Read the model definition and answer for the solid it produces. Units are mm, in the model's axes. A direction names the side the tool comes from. Round coordinates to 2 decimals unless told otherwise and drop trailing zeros. Write each loop counter-clockwise with the first axis right and the second up, starting at its lowest first coordinate (ties: lowest second). Pieces come first, ordered by that corner, then holes. Notation, with made-up numbers: (31.5, 46.25) - (73.5, 46.25) arc R27 cw to (73.5, 81.25) - close; hole circle Ø10 at (43, 33.5). An arc over 180 degrees is marked (long way). Answer as CSV lines item,"result". Start each with the question number.
1) For a pull along Y with two mould halves and no side action, classify faces 4 (the flat face through (-16, -10, 0)), 5 (the flat face through (6.736, 6.267, 1.972)), 6 (the cylindrical face through (-62, 36.12, 17.97)), 7 (the flat face through (-0.946, -35.738, 1.972)) as +Y half, -Y half, draft (parallel to the pull), parting line (faces both ways), or undercut.
2) Find section C-C on x = -38. Determine the outline of the cut face in (y, z).
3) Consider line 1 along X through (y, z) = (17.5, 2.5); line 2 along X through (y, z) = (-19, 1.25); line 3 along X through (y, z) = (-10.5, 5.5). Determine where each line is inside the solid, lowest interval first.
4) Each of these flat-tipped pins is pushed along its axis until it touches: pin 1 (2.5 mm diameter, centred on x = -59.5, y = 28, fed in from -Z); pin 2 (1.5 mm diameter, centred on x = 28, y = 26.5, fed in from -Z); pin 3 (4 mm diameter, centred on x = -25.5, z = 16.5, fed in from -Y); pin 4 (5 mm diameter, centred on x = -11.5, z = 12.5, fed in from -Y). Where does it stop, or does it pass through?
5) Find section A-A on z = 18.5. Determine the outline of the cut face in (x, y), then the cut area to 3 significant figures.
6) Which of the six approach directions +Z, -Z, +X, -X, +Y, -Y give full straight-line access (tool end or side, diameter ignored) to faces 1 (the flat face through (-16, -10, 4)), 2 (the flat face through (-37.234, -32.15, 1.972)), 3 (the flat face through (21, 34, 3))?
7) Find section B-B on z = 7.5. Determine the outline of the cut face in (x, y).
8) Find section D-D on y = -1.5. Determine the outline of the cut face in (x, z), then the cut area to 3 significant figures.
from build123d import *

# Parameters (mm, degrees)
F1_DEPTH  = 4
F3_DEPTH  = 12
F7_DEPTH  = 4
F8_DEPTH  = 25
F9_R      = 2
F10_DEPTH = 25
F12_DEPTH = 4
F13_R     = 1.5
F14_DEPTH = 3


with BuildPart() as f1:
    # F0 (on Top) → F1 (new body)
    with BuildSketch(Plane.XY):
        with BuildLine():
            Line((27.792761, 37.208434), (-59.207239, 37.208434))
            ThreePointArc((-59.207239, 37.208434), (-62.035666, 36.036861), (-63.207239, 33.208434))
            Line((-63.207239, 33.208434), (-63.207239, -53.791566))
            ThreePointArc((-63.207239, -53.791566), (-62.035666, -56.619993), (-59.207239, -57.791566))
            Line((-59.207239, -57.791566), (27.792761, -57.791566))
            ThreePointArc((27.792761, -57.791566), (30.621188, -56.619993), (31.792761, -53.791566))
            Line((31.792761, -53.791566), (31.792761, 33.208434))
            ThreePointArc((31.792761, 33.208434), (30.621188, 36.036861), (27.792761, 37.208434))
        make_face()
    extrude(amount=F1_DEPTH)

    # F2 (on face) → F3 (join)
    with BuildSketch(Plane.XY.offset(4)):
        with BuildLine():
            ThreePointArc((30.792761, -10.291566), (27.253159, 7.503214), (17.173226, 22.5889))
            Line((17.173226, 22.5889), (-15.707239, -10.291566))
            Line((-15.707239, -10.291566), (17.173226, -43.172031))
            ThreePointArc((17.173226, -43.172031), (27.253159, -28.086345), (30.792761, -10.291566))
        make_face()
        with BuildLine():
            Line((-15.707239, -10.291566), (17.173226, 22.5889))
            ThreePointArc((17.173226, 22.5889), (-15.707239, 36.208434), (-48.587704, 22.5889))
            Line((-48.587704, 22.5889), (-15.707239, -10.291566))
        make_face()
        with BuildLine():
            Line((17.173226, -43.172031), (-15.707239, -10.291566))
            Line((-15.707239, -10.291566), (-48.587704, -43.172031))
            ThreePointArc((-48.587704, -43.172031), (-15.707239, -56.791566), (17.173226, -43.172031))
        make_face()
        with BuildLine():
            Line((-48.587704, -43.172031), (-15.707239, -10.291566))
            Line((-15.707239, -10.291566), (-48.587704, 22.5889))
            ThreePointArc((-48.587704, 22.5889), (-62.207239, -10.291566), (-48.587704, -43.172031))
        make_face()
    extrude(amount=F3_DEPTH)

    # F6 (on offset) → F7 (join)
    with BuildSketch(Plane.XY.offset(16)):
        with BuildLine():
            ThreePointArc((-59.207239, 37.256276), (-62.035666, 36.084703), (-63.207239, 33.256276))
            Line((-63.207239, 33.256276), (-63.207239, -53.743724))
            ThreePointArc((-63.207239, -53.743724), (-62.035666, -56.572152), (-59.207239, -57.743724))
            Line((-59.207239, -57.743724), (27.792761, -57.743724))
            ThreePointArc((27.792761, -57.743724), (30.621188, -56.572152), (31.792761, -53.743724))
            Line((31.792761, -53.743724), (31.792761, 33.256276))
            ThreePointArc((31.792761, 33.256276), (30.621188, 36.084703), (27.792761, 37.256276))
            Line((27.792761, 37.256276), (-59.207239, 37.256276))
        make_face()
    extrude(amount=F7_DEPTH)

    # F4 (on face) → F8 (cut)
    with BuildSketch(Plane(origin=(0, 0, 0), x_dir=(1, 0, 0), z_dir=(0, 0, -1))):
        with BuildLine():
            ThreePointArc((16.112566, 42.111371), (-15.707239, 55.291566), (-47.527044, 42.111371))
            Line((-47.527044, 42.111371), (-15.707239, 10.291566))
            Line((-15.707239, 10.291566), (16.112566, 42.111371))
        make_face()
        with BuildLine():
            Line((-15.707239, 10.291566), (-47.527044, 42.111371))
            ThreePointArc((-47.527044, 42.111371), (-60.707239, 10.291566), (-47.527044, -21.528239))
            Line((-47.527044, -21.528239), (-15.707239, 10.291566))
        make_face()
        with BuildLine():
            Line((16.112566, 42.111371), (-15.707239, 10.291566))
            Line((-15.707239, 10.291566), (16.112566, -21.528239))
            ThreePointArc((16.112566, -21.528239), (25.86734, -6.929189), (29.292761, 10.291566))
            ThreePointArc((29.292761, 10.291566), (25.86734, 27.51232), (16.112566, 42.111371))
        make_face()
        with BuildLine():
            Line((16.112566, -21.528239), (-15.707239, 10.291566))
            Line((-15.707239, 10.291566), (-47.527044, -21.528239))
            ThreePointArc((-47.527044, -21.528239), (-15.707239, -34.708434), (16.112566, -21.528239))
        make_face()
    extrude(amount=-F8_DEPTH, mode=Mode.SUBTRACT)

    # F9 (on face) → F10 (cut)
    with BuildSketch(Plane(origin=(0, 0, 0), x_dir=(1, 0, 0), z_dir=(0, 0, -1))):
        with Locations((27.792761, 53.791566)):
            Circle(F9_R)
        with Locations((27.792761, -33.208434)):
            Circle(F9_R)
        with Locations((-59.207239, 53.791566)):
            Circle(F9_R)
        with Locations((-59.207239, -33.208434)):
            Circle(F9_R)
    extrude(amount=-F10_DEPTH, mode=Mode.SUBTRACT)

    # F11 (on Top) → F12 (join)
    with BuildSketch(Plane.XY):
        with BuildLine():
            ThreePointArc((-11.075309, -27.358951), (-7.059758, -25.616863), (-3.602133, -22.932771))
            Line((-3.602133, -22.932771), (-15.977767, -10.559668))
            Line((-15.977767, -10.559668), (-28.343116, -22.94305))
            ThreePointArc((-28.343116, -22.94305), (-22.668837, -26.729999), (-15.977767, -28.059668))
            ThreePointArc((-15.977767, -28.059668), (-13.501626, -27.883603), (-11.075309, -27.358951))
        make_face()
        with BuildLine():
            Line((-15.977767, -10.559668), (-3.602133, -22.932771))
            ThreePointArc((-3.602133, -22.932771), (-0.097014, -17.911653), (1.463653, -11.990353))
            ThreePointArc((1.463653, -11.990353), (1.507582, -11.27561), (1.522233, -10.559668))
            ThreePointArc((1.522233, -10.559668), (1.284893, -7.687292), (0.579313, -4.892827))
            ThreePointArc((0.579313, -4.892827), (-1.131734, -1.294395), (-3.612418, 1.823714))
            Line((-3.612418, 1.823714), (-15.977767, -10.559668))
        make_face()
        with BuildLine():
            Line((-28.343116, -22.94305), (-15.977767, -10.559668))
            Line((-15.977767, -10.559668), (-28.353402, 1.813434))
            ThreePointArc((-28.353402, 1.813434), (-32.406411, -4.530599), (-33.419188, -11.990353))
            ThreePointArc((-33.419188, -11.990353), (-32.996271, -14.636499), (-32.174304, -17.187051))
            ThreePointArc((-32.174304, -17.187051), (-30.545822, -20.256152), (-28.343116, -22.94305))
        make_face()
        with BuildLine():
            Line((-28.353402, 1.813434), (-15.977767, -10.559668))
            Line((-15.977767, -10.559668), (-3.612418, 1.823714))
            ThreePointArc((-3.612418, 1.823714), (-9.286698, 5.610662), (-15.977767, 6.940332))
            ThreePointArc((-15.977767, 6.940332), (-18.453909, 6.764267), (-20.880226, 6.239615))
            ThreePointArc((-20.880226, 6.239615), (-24.895777, 4.497526), (-28.353402, 1.813434))
        make_face()
        with BuildLine():
            Line((17.595724, -42.005187), (-11.075309, -27.358951))
            ThreePointArc((-11.075309, -27.358951), (-13.501626, -27.883603), (-15.977767, -28.059668))
            Line((-15.977767, -28.059668), (15.474621, -44.126725))
            Line((15.474621, -44.126725), (17.595724, -42.005187))
        make_face()
        with BuildLine():
            ThreePointArc((1.522233, -10.559668), (1.507582, -11.27561), (1.463653, -11.990353))
            Line((1.463653, -11.990353), (12.343387, 25.688259))
            Line((12.343387, 25.688259), (9.920419, 27.457222))
            Line((9.920419, 27.457222), (0.579313, -4.892827))
            ThreePointArc((0.579313, -4.892827), (1.284893, -7.687292), (1.522233, -10.559668))
        make_face()
        with BuildLine():
            ThreePointArc((15.474621, -44.126725), (16.552472, -43.083252), (17.595724, -42.005187))
            Line((17.595724, -42.005187), (15.474621, -44.126725))
        make_face()
        with BuildLine():
            Line((9.920419, 27.457222), (12.343387, 25.688259))
            ThreePointArc((12.343387, 25.688259), (11.146328, 26.592498), (9.920419, 27.457222))
        make_face()
        with BuildLine():
            Line((-49.551259, 20.885851), (-20.880226, 6.239615))
            ThreePointArc((-20.880226, 6.239615), (-18.453909, 6.764267), (-15.977767, 6.940332))
            Line((-15.977767, 6.940332), (-47.430156, 23.007388))
            Line((-47.430156, 23.007388), (-49.551259, 20.885851))
        make_face()
        with BuildLine():
            ThreePointArc((-32.174304, -17.187051), (-32.996271, -14.636499), (-33.419188, -11.990353))
            Line((-33.419188, -11.990353), (-45.001782, -46.247293))
            Line((-45.001782, -46.247293), (-42.613842, -48.063262))
            Line((-42.613842, -48.063262), (-32.174304, -17.187051))
        make_face()
        with BuildLine():
            ThreePointArc((-47.430156, 23.007388), (-48.508007, 21.963916), (-49.551259, 20.885851))
            Line((-49.551259, 20.885851), (-47.430156, 23.007388))
        make_face()
        with BuildLine():
            Line((-42.613842, -48.063262), (-45.001782, -46.247293))
            ThreePointArc((-45.001782, -46.247293), (-43.82262, -47.17475), (-42.613842, -48.063262))
        make_face()
    extrude(amount=F12_DEPTH)

    # F13 (on face) → F14 (cut)
    with BuildSketch(Plane(origin=(0, 0, 0), x_dir=(1, 0, 0), z_dir=(0, 0, -1))):
        with Locations((28.893428, 47.575925)):
            Circle(F13_R)
        with Locations((-53.599834, 55.02338)):
            Circle(F13_R)
        with Locations((-60.483862, 47.575925)):
            Circle(F13_R)
        with Locations((27.792761, -27.104519)):
            Circle(F13_R)
        with Locations((-59.352773, -27.413523)):
            Circle(F13_R)
        with Locations((-52.714072, -34.026481)):
            Circle(F13_R)
        with Locations((20.607447, -33.641927)):
            Circle(F13_R)
    extrude(amount=-F14_DEPTH, mode=Mode.SUBTRACT)


solid = f1.part
Check values:
1,face 4,"draft"
1,face 5,"undercut"
1,face 6,"+Y half"
1,face 7,"undercut"
2,outline,"(-57.79, 0) - (-49.38, 0) - (-49.38, 20) - (-57.74, 20) - (-57.74, 16) - (-51.1, 16) - (-51.1, 4) - (-57.79, 4) - close; (-34.42, 0) - (-25.54, 0) - (-25.54, 4) - (-34.42, 4) - close; (14.99, 0) - (18.19, 0) - (18.19, 4) - (14.99, 4) - close; (28.8, 0) - (37.21, 0) - (37.21, 4) - (30.52, 4) - (30.52, 16) - (37.26, 16) - (37.26, 20) - (28.8, 20) - close"
3,line 1,"x = -63.21 to -51.1, -42.92 to -36.65, 7.05 to 9.98, 19.69 to 31.79"
3,line 2,"x = -63.21 to -59.86, -35.79 to -32.79, -31.31 to -0.65, 28.44 to 31.79"
3,line 3,"x = -62.21 to -60.71, 29.29 to 30.79"
4,pin 1,"stops at z = 0"
4,pin 2,"stops at z = 3"
4,pin 3,"stops at y = -57.74"
4,pin 4,"stops at y = -56.76"
5,outline,"(-63.21, -53.74) arc R4 ccw to (-59.21, -57.74) - (27.79, -57.74) arc R4 ccw to (31.79, -53.74) - (31.79, 33.26) arc R4 ccw to (27.79, 37.26) - (-59.21, 37.26) arc R4 ccw to (-63.21, 33.26) - close; hole circle Ø4 at (-59.21, -53.79); hole circle Ø4 at (-59.21, 33.21); hole (-47.53, 21.53) arc R45 ccw to (16.11, -42.11) arc R45 ccw to (29.29, -10.29) arc R45 ccw to (16.11, 21.53) arc R45 ccw to start; hole circle Ø4 at (27.79, -53.79); hole circle Ø4 at (27.79, 33.21)"
5,area,"2,600 mm^2"
6,face 1,"+Z"
6,face 2,"+Z, -Z"
6,face 3,"-Z"
7,outline,"(-48.59, -43.17) arc R46.5 ccw to (17.17, -43.17) arc R46.5 ccw to (30.79, -10.29) arc R46.5 ccw to (17.17, 22.59) arc R46.5 ccw to (-48.59, 22.59) arc R46.5 ccw to start; hole (-47.53, 21.53) arc R45 ccw to (16.11, -42.11) arc R45 ccw to (29.29, -10.29) arc R45 ccw to (16.11, 21.53) arc R45 ccw to start"
8,outline,"(-63.21, 0) - (-59.84, 0) - (-59.84, 20) - (-63.21, 20) - (-63.21, 16) - (-61.37, 16) - (-61.37, 4) - (-63.21, 4) - close; (-30.95, 0) - (-1.01, 0) - (-1.01, 4) - (-30.95, 4) - close; (1.56, 0) - (4.49, 0) - (4.49, 4) - (1.56, 4) - close; (28.43, 0) - (31.79, 0) - (31.79, 4) - (29.95, 4) - (29.95, 16) - (31.79, 16) - (31.79, 20) - (28.43, 20) - close"
8,area,"222 mm^2"
